Geometry check sheet. Reference: the model listing, model coordinates, mm. Face numbers are marked on the shaded views. A direction names the side the tool comes from. Coordinates: 2 decimals unless noted, no trailing zeros. Write each loop counter-clockwise with the first axis right and the second up, starting at its lowest first coordinate (ties: lowest second). Pieces come first, ordered by that corner, then holes. Notation, with made-up numbers: (27.5, 79) -> (80.5, 79) arc R24 ccw to (80.5, 105) -> close; hole circle Ø10 at (28, -23.5). An arc over 180 degrees is marked (long way). Answer in a Markdown table with one row per item. Add a question column.
Q1. Gauge pin test, flat ends, axial feed: P1, Ø0.9, axis at y = -6.5, z = 4, coming from the +X side; P2, Ø2.5, axis at x = 7.5, y = 14.5, coming from the -Z side; P3, Ø3, axis at x = -1.5, y = -1.5, coming from the +Z side. Record the tip position at first contact, or that the pin passes through.
Q2. Tool access check on the marked faces 3, 4, 5, 6 and 7. Record the directions out of +Z, -Z, +X, -X, +Y, -Y that give a thin tool (end or side, any length) a straight path to the whole face; none if there is none.
Q3. Section check D-D, the plane z = 0.5. Record the boundary of the cut face in (x, y).
Q4. Section check C-C, the plane z = 3.5. Count the separate pieces of the cut face and the enclosed holes in it, and give its area (3 significant figures).
Q5. Section check B-B, the plane y = 13. Record the boundary of the cut face in (x, z), and give its area (3 significant figures).
Q6. Thickness scan on line 1 (Y direction, x = 0, z = 0.9); line 2 (X direction, y = -14, z = 3.25); line 3 (Z direction, x = -9, y = -16.6). Record the ranges inside material, lowest first.
Q7. Release check for a two-part mould opening along Y. For the marked faces 1 and 2 record: pulls with the +Y half, pulls with the -Y half, needs draft (parallel to the pull), parting line crosses it, or undercut.
Q8. Section check A-A, the plane x = 0. Record the boundary of the cut face in (y, z).
```python
from build123d import *

# Parameters (mm, degrees)
SKETCH_1_R          = 11
EXTRUDE_1_DEPTH     = 2
EXTRUDE_2_DEPTH     = 3
SKETCH_4_R          = 0.9
CUT_EXTRUDE_1_DEPTH = 4
SKETCH_5_R          = 0.9
CUT_EXTRUDE_2_DEPTH = 4
SKETCH_6_R          = 0.9
CUT_EXTRUDE_3_DEPTH = 4
SKETCH_8_R          = 11
EXTRUDE_3_DEPTH     = 3
SKETCH_9_R          = 4.723532035
CUT_EXTRUDE_4_DEPTH = 2


with BuildPart() as part:
    # 草图1 → 凸台-拉伸1 (new body)
    with BuildSketch(Plane.XY):
        Circle(SKETCH_1_R)
    extrude(amount=EXTRUDE_1_DEPTH)

    # 草图2 → 凸台-拉伸2 (add)
    with BuildSketch(Plane.XY.offset(2)):
        with BuildLine():
            ThreePointArc((-5.674338907, 9.423474835), (-6.722663515, 8.706652357), (-7.681381188, 7.873778194))
            Line((-7.681381188, 7.873778194), (-2.2295398, 4.726156102))
            Line((-2.2295398, 4.726156102), (-1.056740901, 6.757503383))
            Line((-1.056740901, 6.757503383), (-5.674338907, 9.423474835))
        make_face()
        with BuildLine():
            Line((-11, 19.052558883), (-13, 15.588457268))
            ThreePointArc((-13, 15.588457268), (-8.322973179, 13.122163256), (-7.681381188, 7.873778194))
            ThreePointArc((-7.681381188, 7.873778194), (-6.722663515, 8.706652357), (-5.674338907, 9.423474835))
            ThreePointArc((-5.674338907, 9.423474835), (-5.965261919, 15.549873274), (-11, 19.052558883))
        make_face()
        with BuildLine():
            Line((-20, 3.464101615), (-22, 0))
            ThreePointArc((-22, 0), (-16.44921624, -2.608868275), (-10.998138053, 0.202384226))
            ThreePointArc((-10.998138053, 0.202384226), (-10.901513881, 1.468671206), (-10.659582534, 2.715382148))
            ThreePointArc((-10.659582534, 2.715382148), (-15.525613322, 0.64682458), (-20, 3.464101615))
        make_face()
        with BuildLine():
            ThreePointArc((-10.659582534, 2.715382148), (-10.901513881, 1.468671206), (-10.998138053, 0.202384226))
            Line((-10.998138053, 0.202384226), (-6.380540046, -2.463587226))
            Line((-6.380540046, -2.463587226), (-5.207741146, -0.432239945))
            Line((-5.207741146, -0.432239945), (-10.659582534, 2.715382148))
        make_face()
        with BuildLine():
            ThreePointArc((-5.323799145, -9.625859061), (-10.483954321, -12.941004999), (-11, -19.052558883))
            Line((-11, -19.052558883), (-7, -19.052558883))
            ThreePointArc((-7, -19.052558883), (-7.202640143, -13.768987836), (-2.978201346, -10.589160342))
            ThreePointArc((-2.978201346, -10.589160342), (-4.178850366, -10.175323563), (-5.323799145, -9.625859061))
        make_face()
        with BuildLine():
            Line((-5.323799145, -4.293916157), (-5.323799145, -9.625859061))
            ThreePointArc((-5.323799145, -9.625859061), (-4.178850366, -10.175323563), (-2.978201346, -10.589160342))
            Line((-2.978201346, -10.589160342), (-2.978201346, -4.293916157))
            Line((-2.978201346, -4.293916157), (-5.323799145, -4.293916157))
        make_face()
        with BuildLine():
            Line((2.978201346, -4.293916157), (2.978201346, -10.589160342))
            ThreePointArc((2.978201346, -10.589160342), (4.178850366, -10.175323563), (5.323799145, -9.625859061))
            Line((5.323799145, -9.625859061), (5.323799145, -4.293916157))
            Line((5.323799145, -4.293916157), (2.978201346, -4.293916157))
        make_face()
        with BuildLine():
            ThreePointArc((2.978201346, -10.589160342), (7.202640143, -13.768987836), (7, -19.052558883))
            Line((7, -19.052558883), (11, -19.052558883))
            ThreePointArc((11, -19.052558883), (10.483954321, -12.941004999), (5.323799145, -9.625859061))
            ThreePointArc((5.323799145, -9.625859061), (4.178850366, -10.175323563), (2.978201346, -10.589160342))
        make_face()
        with BuildLine():
            ThreePointArc((10.998138053, 0.202384226), (16.44921624, -2.608868275), (22, 0))
            Line((22, 0), (20, 3.464101615))
            ThreePointArc((20, 3.464101615), (15.525613322, 0.64682458), (10.659582534, 2.715382148))
            ThreePointArc((10.659582534, 2.715382148), (10.901513881, 1.468671206), (10.998138053, 0.202384226))
        make_face()
        with BuildLine():
            Line((6.380540046, -2.463587226), (10.998138053, 0.202384226))
            ThreePointArc((10.998138053, 0.202384226), (10.901513881, 1.468671206), (10.659582534, 2.715382148))
            Line((10.659582534, 2.715382148), (5.207741146, -0.432239945))
            Line((5.207741146, -0.432239945), (6.380540046, -2.463587226))
        make_face()
        with BuildLine():
            ThreePointArc((7.681381188, 7.873778194), (6.722663515, 8.706652357), (5.674338907, 9.423474835))
            Line((5.674338907, 9.423474835), (1.056740901, 6.757503383))
            Line((1.056740901, 6.757503383), (2.2295398, 4.726156102))
            Line((2.2295398, 4.726156102), (7.681381188, 7.873778194))
        make_face()
        with BuildLine():
            Line((13, 15.588457268), (11, 19.052558883))
            ThreePointArc((11, 19.052558883), (5.965261919, 15.549873274), (5.674338907, 9.423474835))
            ThreePointArc((5.674338907, 9.423474835), (6.722663515, 8.706652357), (7.681381188, 7.873778194))
            ThreePointArc((7.681381188, 7.873778194), (8.322973179, 13.122163256), (13, 15.588457268))
        make_face()
    extrude(amount=EXTRUDE_2_DEPTH)

    # 草图4 → 切除-拉伸1 (cut)
    with BuildSketch(Plane(origin=(-16.5, 9.526279442, 0), x_dir=(0, 0, 1), z_dir=(-0.866025404, 0.5, 0))):
        with Locations((3.5, 9)):
            Circle(SKETCH_4_R)
        with Locations((3.5, -9)):
            Circle(SKETCH_4_R)
    extrude(amount=-CUT_EXTRUDE_1_DEPTH, mode=Mode.SUBTRACT)

    # 草图5 → 切除-拉伸2 (cut)
    with BuildSketch(Plane(origin=(16.5, 9.526279442, 0), x_dir=(0, 0, -1), z_dir=(0.866025404, 0.5, 0))):
        with Locations((-3.5, -9)):
            Circle(SKETCH_5_R)
        with Locations((-3.5, 9)):
            Circle(SKETCH_5_R)
    extrude(amount=-CUT_EXTRUDE_2_DEPTH, mode=Mode.SUBTRACT)

    # 草图6 → 切除-拉伸3 (cut)
    with BuildSketch(Plane.XZ.offset(19.052558883)):
        with Locations((-9, 3.5)):
            Circle(SKETCH_6_R)
        with Locations((9, 3.5)):
            Circle(SKETCH_6_R)
    extrude(amount=-CUT_EXTRUDE_3_DEPTH, mode=Mode.SUBTRACT)

    # 草图8 → 凸台-拉伸3 (add)
    with BuildSketch(Plane(origin=(0, 0, 0), x_dir=(-1, 0, 0), z_dir=(0, 0, -1))):
        Circle(SKETCH_8_R)
    extrude(amount=EXTRUDE_3_DEPTH)

    # 草图9 → 切除-拉伸4 (cut)
    with BuildSketch(Plane.XY.offset(2)):
        Circle(SKETCH_9_R)
    extrude(amount=-CUT_EXTRUDE_4_DEPTH, mode=Mode.SUBTRACT)


solid = part.part
```
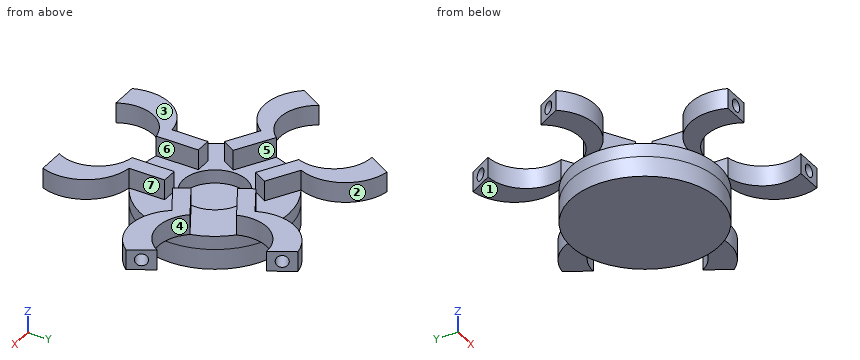
Calculated:
| question | item | result |
|---|---|---|
| 1 | P1 | stops at x = 5.32 |
| 1 | P2 | stops at z = 2 |
| 1 | P3 | stops at z = 0 |
| 2 | face 3 | +Z, +X, -X, +Y, -Y |
| 2 | face 4 | +Z, -Z |
| 2 | face 5 | +Z |
| 2 | face 6 | +Z, -Y |
| 2 | face 7 | +Z, +X |
| 3 | outline | circle Ø22 at (0, 0); hole circle Ø9.45 at (0, 0) |
| 4 | separate pieces | 6 |
| 4 | enclosed holes | 0 |
| 4 | area | 251 mm² |
| 5 | outline | (-8.24, 2) -> (-5.15, 2) -> (-5.15, 5) -> (-8.24, 5) -> close; (5.15, 2) -> (8.24, 2) -> (8.24, 5) -> (5.15, 5) -> close |
| 5 | area | 18.6 mm² |
| 6 | line 1 | y = -11 to -4.72, 4.72 to 11 |
| 6 | line 2 | x = -11 to -7.31, 7.31 to 11 |
| 6 | line 3 | z = 2 to 2.6, 4.4 to 5 |
| 7 | face 1 | needs draft |
| 7 | face 2 | undercut |
| 8 | outline | (-11, -3) -> (11, -3) -> (11, 2) -> (4.72, 2) -> (4.72, 0) -> (-4.72, 0) -> (-4.72, 2) -> (-11, 2) -> close |
